from build123d import *

# Parameters (mm, degrees)
SKETCH1_W           = 40.3
SKETCH1_H           = 40.3
BOSS_EXTRUDE1_DEPTH = 3.7
SKETCH3_R           = 0.85
BOSS_EXTRUDE2_DEPTH = 0.5
SKETCH5_R           = 0.85
SKETCH6_R           = 0.85
BOSS_EXTRUDE3_DEPTH = 10.5


with BuildPart() as part:
    # Sketch1 → Boss-Extrude1 (new body)
    with BuildSketch(Plane(origin=(0, 0, 0), x_dir=(1, 0, 0), z_dir=(0, 1, 0))):
        Rectangle(SKETCH1_W, SKETCH1_H)
    extrude(amount=BOSS_EXTRUDE1_DEPTH)

    # Sketch3 → Boss-Extrude2 (add)
    with BuildSketch(Plane.XY.offset(20.15)):
        with Locations((-17.7, 1.85)):
            Circle(SKETCH3_R)
    boss_extrude2 = extrude(amount=BOSS_EXTRUDE2_DEPTH)

    # Sweep1: sweep along a path in Sketch4
    with BuildLine(Plane.ZY.offset(17.7)) as sweep1_path:
        ThreePointArc((20.65, 1.85), (21.842957341, 2.359410226), (22.3, 3.573394576))
    # Sketch5 → Sweep1 (sweep)
    with BuildSketch(Plane.XY.offset(20.65)):
        with Locations((-17.7, 1.85)):
            Circle(SKETCH5_R)
    sweep1 = sweep(path=sweep1_path.line)

    # Sketch6 → Boss-Extrude3 (add)
    with BuildSketch(Plane(origin=(0, 2.597654528, -0.113087301), x_dir=(1, 0, 0), z_dir=(0, 0.999053723, -0.043493193))):
        with Locations((-17.7, -22.434316371)):
            Circle(SKETCH6_R)
    boss_extrude3 = extrude(amount=BOSS_EXTRUDE3_DEPTH)

    # Mirror1: Boss-Extrude2, Sweep1, Boss-Extrude3 across plane
    add(boss_extrude2.mirror(Plane(origin=(0, 0, 0), x_dir=(0, 0, 1), z_dir=(1, 0, 0))))
    add(sweep1.mirror(Plane(origin=(0, 0, 0), x_dir=(0, 0, 1), z_dir=(1, 0, 0))))
    add(boss_extrude3.mirror(Plane(origin=(0, 0, 0), x_dir=(0, 0, 1), z_dir=(1, 0, 0))))


solid = part.part
The listing builds one solid part. Answer for the finished solid, in the listing's coordinates (mm). A direction names the side the tool comes from. Give positions to 0.01 mm unless a question says otherwise; leave off trailing zeros. Loops run counter-clockwise (first coordinate to the right, second up) from the corner with the lowest first, then second, coordinate; pieces in that order, holes last. Notation, with made-up numbers: (18.25, -10) - (65.25, -10) arc R23 cw to (65.25, -2) - close; hole circle Ø8 at (-28.75, 82). An arc over 180 degrees is marked (long way). Answer as a JSON object with one key per item and string values.
1. For faces 1 (the cylindrical face through (18.55, 1.89, 20.4)), 2 (the flat face through (0, 0, 0)), determine the directions among +Z, -Z, +X, -X, +Y, -Y from which every point of the face is accessible in a straight line to the end or side of a thin tool.
Determined:
{"face 1": "none", "face 2": "+Z, -Z, +X, -X, -Y"}
2. Find the intervals of material crossed by L1, parallel to Y at x = 18.5, z = 12; L2, parallel to Z at x = -15, y = 1.25; L3, parallel to Z at x = -17, y = 5.5, in increasing order. Write a range as [from, to].
Determined:
{"L1": "[0, 3.7]", "L2": "[-20.15, 20.15]", "L3": "[21.73, 22.7]"}
3. Flat-ended cylindrical pins translate along their axes: pin 1 Ø4 at (x, y) = (-2, 2) entering from +Z; pin 2 Ø5 at (y, z) = (8, 10.5) entering from +X; pin 3 Ø2 at (x, z) = (14.5, 2.5) entering from +Y. Find the tip coordinate at first contact, or state that the pin passes through.
Determined:
{"pin 1": "z = 20.15", "pin 2": "through", "pin 3": "y = 3.7"}
4. A cutting plane is placed at B-B (z = 17.5). Write down the section's boundary in (x, y).
Determined:
{"outline": "(-20.15, 0) - (20.15, 0) - (20.15, 3.7) - (-20.15, 3.7) - close"}
5. For a pull along X with two mould halves and no side action, classify faces 3 (the cylindrical face through (-18.55, 8.74, 22.04)), 4 (the flat face through (-20.15, 2, 0)), 5 (the flat face through (0, 3.7, 0)), 6 (the flat face through (0, 2, 20.15)) as pulls with the +X half, pulls with the -X half, needs draft (parallel to the pull), parting line crosses it, or undercut.
Determined:
{"face 3": "undercut", "face 4": "pulls with the -X half", "face 5": "needs draft", "face 6": "undercut"}
6. A cutting plane is placed at C-C (x = -7). Write down the section's boundary in (y, z), then the cut area to 3 significant figures.
Determined:
{"outline": "(0, -20.15) - (3.7, -20.15) - (3.7, 20.15) - (0, 20.15) - close", "area": "149 mm²"}
7. A cutting plane is placed at A-A (x = 17.7). Write down the section's boundary in (y, z), then the cut area to 3 significant figures.
Determined:
{"outline": "(0, -20.15) - (3.7, -20.15) - (3.7, 20.15) - (2.7, 20.15) - (2.7, 20.65) arc R0.8 cw to (3.54, 21.45) - (14.03, 20.99) - (14.1, 22.69) - (3.61, 23.15) arc R2.5 ccw to (1, 20.65) - (1, 20.15) - (0, 20.15) - close", "area": "172 mm²"}
